Verification items for the finished model (mm, model axes). Give positions to 0.01 mm unless a question says otherwise; leave off trailing zeros. Use one line per item in the form item = value. Start each with the question number.
(1) Section check A-A, the plane y = 2.75. State how many separate pieces and enclosed holes the cut face has, plus the area to 3 significant figures.
(2) Scan lines: L1, parallel to X at y = 4, z = -0.5; L2, parallel to X at y = 5.25, z = -21.5; L3, parallel to X at y = 5.75, z = 1. Record each from-to range of solid material in increasing order.
(3) Depth check by flat-ended pin: pin 1 Ø1.8 at (x, z) = (79.25, 23.54) entering from -Y; pin 2 Ø3 at (x, y) = (98.5, 4.5) entering from -Z (3 decimals); pin 3 Ø0.8 at (y, z) = (4, 24.5) entering from -X; pin 4 Ø1.9 at (y, z) = (3.5, -26.5) entering from +X. Enter the tip coordinate at first touch or a pass-through.
from build123d import *

# Parameters (mm, degrees)
BOSS_EXTRUDE1_DEPTH = 6.35
SKETCH2_R           = 1.1303
CUT_EXTRUDE1_DEPTH  = 10.16
SKETCH3_R           = 5.08
SKETCH3_W           = 3.048
SKETCH3_H           = 1.524
CUT_EXTRUDE2_DEPTH  = 10.16
SKETCH4_R           = 1.1303
CUT_EXTRUDE3_DEPTH  = 10.16
SKETCH5_W           = 16.51
SKETCH5_H           = 19.05
CUT_EXTRUDE4_DEPTH  = 10.16


with BuildPart() as part:
    # Sketch1 → Boss-Extrude1 (new body)
    with BuildSketch(Plane(origin=(0, 0, 0), x_dir=(1, 0, 0), z_dir=(0, 1, 0))):
        Polygon((-95.504, 15.875), (-101.6, 15.875), (-101.6, -15.875), (-95.504, -15.875), (-95.504, -33.02), (-70.104, -33.02), (-70.104, -19.812), (-63.5, -19.812), (-63.5, -33.02), (2.794, -33.02), (9.398, -33.02), (62.484, -33.02), (62.484, -19.812), (69.088, -19.812), (69.088, -33.02), (94.488, -33.02), (94.488, -15.875), (100.584, -15.875), (100.584, 15.875), (94.488, 15.875), (94.488, 33.02), (69.088, 33.02), (69.088, 19.812), (62.484, 19.812), (62.484, 33.02), (9.398, 33.02), (2.794, 33.02), (-63.5, 33.02), (-63.5, 19.812), (-70.104, 19.812), (-70.104, 33.02), (-95.504, 33.02), align=None)
    extrude(amount=BOSS_EXTRUDE1_DEPTH)

    # Sketch2 → Cut-Extrude1 (cut)
    with BuildSketch(Plane(origin=(0, 6.35, 0), x_dir=(1, 0, 0), z_dir=(0, 1, 0))):
        with Locations(Location((-5.842, 7.9375, 0), (0, 0, 270))):
            Circle(SKETCH2_R)
        with Locations(Location((4.826, 7.9375, 0), (0, 0, 270))):
            Circle(SKETCH2_R)
        with Locations(Location((4.826, -7.9375, 0), (0, 0, 270))):
            Circle(SKETCH2_R)
        with Locations(Location((-5.842, -7.9375, 0), (0, 0, 270))):
            Circle(SKETCH2_R)
        with Locations(Location((-75.184, 0, 0), (0, 0, 270))):
            Circle(SKETCH2_R)
        with Locations(Location((-24.384, 0, 0), (0, 0, 270))):
            Circle(SKETCH2_R)
        with Locations(Location((43.434, 20.32, 0), (0, 0, 270))):
            Circle(SKETCH2_R)
        with Locations(Location((75.184, 20.32, 0), (0, 0, 270))):
            Circle(SKETCH2_R)
        with Locations(Location((75.184, 6.35, 0), (0, 0, 270))):
            Circle(SKETCH2_R)
        with Locations(Location((43.434, 6.35, 0), (0, 0, 270))):
            Circle(SKETCH2_R)
        with Locations(Location((38.608, -10.839373847, 0), (0, 0, 270))):
            Circle(SKETCH2_R)
        with Locations(Location((79.248, -11.389700319, 0), (0, 0, 270))):
            Circle(SKETCH2_R)
        with Locations(Location((38.608, -23.539373847, 0), (0, 0, 270))):
            Circle(SKETCH2_R)
        with Locations(Location((79.248, -23.539373847, 0), (0, 0, 270))):
            Circle(SKETCH2_R)
    extrude(amount=-CUT_EXTRUDE1_DEPTH, mode=Mode.SUBTRACT)

    # Sketch3 → Cut-Extrude2 (cut)
    with BuildSketch(Plane(origin=(0, 6.35, 0), x_dir=(1, 0, 0), z_dir=(0, 1, 0))):
        with Locations(Location((18.796, 17.78, 0), (0, 0, 270))):
            Circle(SKETCH3_R)
        with Locations((-49.276, 29.718)):
            Rectangle(SKETCH3_W, SKETCH3_H)
        with Locations((-49.276, 24.384)):
            Rectangle(SKETCH3_W, SKETCH3_H)
        with Locations((48.26, 29.718)):
            Rectangle(SKETCH3_W, SKETCH3_H)
        with Locations((48.26, 24.384)):
            Rectangle(SKETCH3_W, SKETCH3_H)
        with Locations((-49.276, -24.384)):
            Rectangle(SKETCH3_W, SKETCH3_H)
        with Locations((-49.276, -29.718)):
            Rectangle(SKETCH3_W, SKETCH3_H)
        with Locations((48.26, -24.384)):
            Rectangle(SKETCH3_W, SKETCH3_H)
        with Locations((48.26, -29.718)):
            Rectangle(SKETCH3_W, SKETCH3_H)
    extrude(amount=-CUT_EXTRUDE2_DEPTH, mode=Mode.SUBTRACT)

    # Sketch4 → Cut-Extrude3 (cut)
    with BuildSketch(Plane(origin=(0, 6.35, 0), x_dir=(1, 0, 0), z_dir=(0, 1, 0))):
        with Locations(Location((-38.1, 26.67, 0), (0, 0, 270))):
            Circle(SKETCH4_R)
        with Locations(Location((32.004, 26.67, 0), (0, 0, 270))):
            Circle(SKETCH4_R)
        with Locations(Location((-38.1, -26.67, 0), (0, 0, 270))):
            Circle(SKETCH4_R)
        with Locations(Location((32.004, -26.67, 0), (0, 0, 270))):
            Circle(SKETCH4_R)
    extrude(amount=-CUT_EXTRUDE3_DEPTH, mode=Mode.SUBTRACT)

    # Sketch5 → Cut-Extrude4 (cut)
    with BuildSketch(Plane(origin=(0, 6.35, 0), x_dir=(1, 0, 0), z_dir=(0, 1, 0))):
        with Locations((-93.345, 0)):
            Rectangle(SKETCH5_W, SKETCH5_H)
        with Locations((92.329, 0)):
            Rectangle(SKETCH5_W, SKETCH5_H)
    extrude(amount=-CUT_EXTRUDE4_DEPTH, mode=Mode.SUBTRACT)


solid = part.part
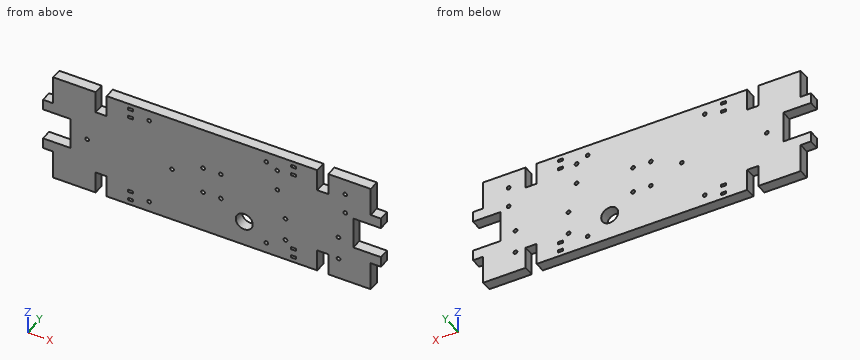
Completed:
q1.separate_pieces = 1
q1.enclosed_holes = 27
q1.area = 11,800 mm²
q2.L1 = -85.09 to -76.2, -74.17 to -25.4, -23.37 to 84.07
q2.L2 = -95.5 to -70.1, -63.5 to 15.34, 22.26 to 62.48, 69.09 to 94.49
q2.L3 = -85.09 to -75.71, -74.66 to -24.91, -23.86 to 84.07
q3.pin_1 = through
q3.pin_2 = -15.875
q3.pin_3 = -95.5
q3.pin_4 = 94.49
